Autodesk Inventor part; units mm, degrees
ref_plane "YZ Plane" through (0, 0, 0) normal (1, 0, 0) x (0, 1, 0)
ref_plane "XZ Plane" through (0, 0, 0) normal (0, 1, 0) x (-1, 0, 0)
ref_plane "XY Plane" through (0, 0, 0) normal (0, 0, 1) x (1, 0, 0)
sketch "Sketch1" plane through (0, 0, 0) normal (0, 1, 0) x (-1, 0, 0)
  line L0 (0, 0) -> (0, -110)
  line L1 (0, -110) -> (56.8, -110)
  line L2 (56.8, -110) -> (56.8, 0)
  line L3 (56.8, 0) -> (0, 0)
  dimension "d0" = 110
  dimension "d1" = 56.8
extrude "Extrusion1" add sketch "Sketch1" along normal blind 2
chamfer "Chamfer1" distance 1.5 angle 45 1 edges at (0, 0, -55)
chamfer "Chamfer2" distance 1.5 angle 45 1 edges at (-56.8, 0, -55)
chamfer "Chamfer3" distance 1.5 angle 45 2 edges at (-28.4, 0, 0) (-28.4, 0, -110)
properties part number "priklop"
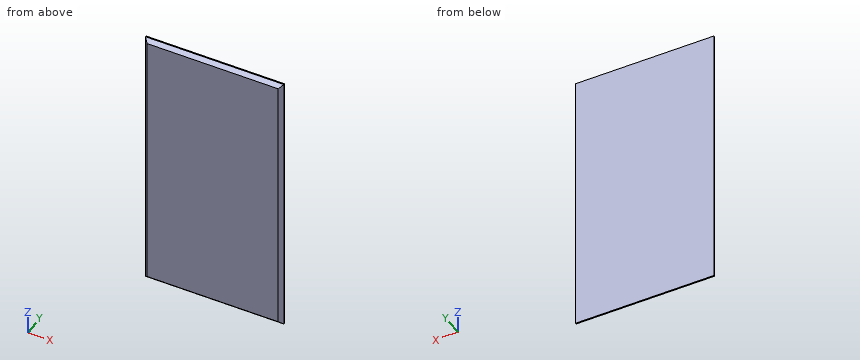
The model under review builds one solid part; all positions refer to its coordinate system, in mm. Round coordinates to 2 decimals unless told otherwise and drop trailing zeros. Loops run counter-clockwise (first coordinate to the right, second up) from the corner with the lowest first, then second, coordinate; pieces in that order, holes last. Notation, with made-up numbers: (-29, 44.5) -> (-1, 44.5) arc R14 cw to (-1, 68.5) -> close; hole circle Ø11 at (42, 48). An arc over 180 degrees is marked (long way). Return JSON: item names as keys, results as strings.
(1) Add section A-A on z = -97.5. Write out the cut boundary in (x, y).
Solved:
{"outline": "(-56.8, 1.5) -> (-55.3, 0) -> (-1.5, 0) -> (0, 1.5) -> (0, 2) -> (-56.8, 2) -> close"}
(2) Add section B-B on y = 0.7. Write out the cut boundary in (x, z).
Solved:
{"outline": "(-56, -109.2) -> (-0.8, -109.2) -> (-0.8, -0.8) -> (-56, -0.8) -> close"}
(3) For line 1 (Z direction, x = -48, y = 1); line 2 (X direction, y = 0.9, z = -42); line 3 (X direction, y = 1.05, z = -14.5), list the stretches that pass through material, from the lowest coordinate up.
Solved:
{"line 1": "-109.5 to -0.5", "line 2": "-56.2 to -0.6", "line 3": "-56.35 to -0.45"}
